```python
from build123d import *

# Parameters (mm, degrees)
SKETCH1_W            = 93
SKETCH1_H            = 100
BOSS_EXTRUDE2_DEPTH  = 10
SKETCH4_W            = 10.01
SKETCH4_H            = 15
BOSS_EXTRUDE4_DEPTH  = 24
SKETCH5_R            = 2
CUT_EXTRUDE1_DEPTH   = 50
SKETCH7_R            = 11
CUT_EXTRUDE3_DEPTH   = 50
SKETCH14_W           = 61.5
SKETCH14_H           = 42
CUT_EXTRUDE8_DEPTH   = 4
SKETCH19_R           = 11
CUT_EXTRUDE11_DEPTH  = 15
SKETCH20_R           = 2
CUT_EXTRUDE12_DEPTH  = 10
SKETCH21_W           = 40
SKETCH21_H           = 6
BOSS_EXTRUDE5_DEPTH  = 27
SKETCH22_W           = 40
SKETCH22_H           = 6.3
BOSS_EXTRUDE7_DEPTH  = 40
SKETCH23_R           = 8
CUT_EXTRUDE13_DEPTH  = 40
SKETCH24_W           = 118.277817783
SKETCH24_H           = 41.8
CUT_EXTRUDE14_DEPTH  = 40
SKETCH25_W           = 31.5
SKETCH25_H           = 23.2
CUT_EXTRUDE15_DEPTH  = 20
CUT_EXTRUDE18_DEPTH  = 3
SKETCH27_R           = 4.1
SKETCH27_R_2         = 4
CUT_EXTRUDE29_DEPTH  = 3
SKETCH28_W           = 29.5
SKETCH28_H           = 58.2
CUT_EXTRUDE30_DEPTH  = 23
SKETCH29_W           = 32
SKETCH29_H           = 4
CUT_EXTRUDE31_DEPTH  = 23
SKETCH31_W           = 32
SKETCH31_H           = 6
BOSS_EXTRUDE9_DEPTH  = 6.6
SKETCH32_W           = 32
SKETCH32_H           = 6
BOSS_EXTRUDE10_DEPTH = 10
SKETCH33_R           = 2
CUT_EXTRUDE32_DEPTH  = 10
BOSS_EXTRUDE11_START = -32
BOSS_EXTRUDE11_DEPTH = 32
SKETCH35_R           = 3.5
CUT_EXTRUDE33_DEPTH  = 10
SKETCH36_W           = 40
SKETCH36_H           = 6.3
BOSS_EXTRUDE12_DEPTH = 18.8
SKETCH37_W           = 40
SKETCH37_H           = 6
BOSS_EXTRUDE13_DEPTH = 16
SKETCH38_R           = 2
CUT_EXTRUDE34_DEPTH  = 16
BOSS_EXTRUDE14_DEPTH = 40
SKETCH40_R           = 3.5
CUT_EXTRUDE35_DEPTH  = 16
SKETCH41_W           = 16
SKETCH41_H           = 64.8
CUT_EXTRUDE36_DEPTH  = 76
SKETCH42_W           = 20.7
SKETCH42_H           = 6
CUT_EXTRUDE37_DEPTH  = 76
SKETCH43_W           = 10.32098901
SKETCH43_H           = 73.075116481
CUT_EXTRUDE38_DEPTH  = 30
SKETCH44_W           = 2
SKETCH44_H           = 70.783229749
CUT_EXTRUDE39_DEPTH  = 30
SKETCH45_W           = 27.67901099
SKETCH45_H           = 15
CUT_EXTRUDE40_DEPTH  = 30
SKETCH46_W           = 27.67901099
SKETCH46_H           = 2.54
CUT_EXTRUDE41_DEPTH  = 110
SKETCH47_R           = 11
CUT_EXTRUDE42_DEPTH  = 20
BOSS_EXTRUDE16_DEPTH = 2.3


with BuildPart() as part:
    # Sketch1 → Boss-Extrude2 (new body)
    with BuildSketch(Plane.XY):
        with Locations((-29.68705036, 14.928057554)):
            Rectangle(SKETCH1_W, SKETCH1_H)
    extrude(amount=BOSS_EXTRUDE2_DEPTH)

    # Sketch4 → Boss-Extrude4 (add)
    with BuildSketch(Plane(origin=(16.81294964, 0, 0), x_dir=(0, 0, -1), z_dir=(1, 0, 0))):
        with Locations((-4.995, -12.571942446)):
            Rectangle(SKETCH4_W, SKETCH4_H)
    extrude(amount=BOSS_EXTRUDE4_DEPTH)

    # Sketch5 → Cut-Extrude1 (cut)
    with BuildSketch(Plane(origin=(0, -5.071942446, 0), x_dir=(1, 0, 0), z_dir=(0, 1, 0))):
        with Locations(Location((26.81294964, -5, 0), (0, 0, 180))):
            Circle(SKETCH5_R)
    extrude(amount=-CUT_EXTRUDE1_DEPTH, mode=Mode.SUBTRACT)

    # Sketch7 → Cut-Extrude3 (cut)
    with BuildSketch(Plane(origin=(0, 0, 0), x_dir=(-1, 0, 0), z_dir=(0, 0, -1))):
        with Locations((24.18705036, 36.928057554)):
            Circle(SKETCH7_R)
    extrude(amount=-CUT_EXTRUDE3_DEPTH, mode=Mode.SUBTRACT)

    # Sketch14 → Cut-Extrude8 (cut)
    with BuildSketch(Plane.XY.offset(10)):
        with Locations((-13.93705036, 36.789132279)):
            Rectangle(SKETCH14_W, SKETCH14_H)
    extrude(amount=-CUT_EXTRUDE8_DEPTH, mode=Mode.SUBTRACT)

    # Sketch19 → Cut-Extrude11 (cut)
    with BuildSketch(Plane(origin=(0, 0, 0), x_dir=(-1, 0, 0), z_dir=(0, 0, -1))):
        with Locations((53.18705036, 36.928057554)):
            Circle(SKETCH19_R)
    extrude(amount=-CUT_EXTRUDE11_DEPTH, mode=Mode.SUBTRACT)

    # Sketch20 → Cut-Extrude12 (cut)
    with BuildSketch(Plane.XY.offset(6)):
        with Locations((-34.68705036, 50.928057554)):
            Circle(SKETCH20_R)
        with Locations((5.31294964, 50.928057554)):
            Circle(SKETCH20_R)
        with Locations((-34.68705036, 22.928057554)):
            Circle(SKETCH20_R)
        with Locations((5.31294964, 22.928057554)):
            Circle(SKETCH20_R)
    extrude(amount=-CUT_EXTRUDE12_DEPTH, mode=Mode.SUBTRACT)

    # Sketch21 → Boss-Extrude5 (add)
    with BuildSketch(Plane(origin=(0, 0, 0), x_dir=(-1, 0, 0), z_dir=(0, 0, -1))):
        with Locations((56.18705036, 61.928057554)):
            Rectangle(SKETCH21_W, SKETCH21_H)
    extrude(amount=BOSS_EXTRUDE5_DEPTH)

    # Sketch22 → Boss-Extrude7 (add)
    with BuildSketch(Plane.XZ.offset(-58.928057554)):
        with Locations((-56.18705036, -23.85)):
            Rectangle(SKETCH22_W, SKETCH22_H)
    extrude(amount=BOSS_EXTRUDE7_DEPTH)

    # Sketch23 → Cut-Extrude13 (cut)
    with BuildSketch(Plane.XY.offset(10)):
        with Locations((-53.18705036, 36.928057554)):
            Circle(SKETCH23_R)
    extrude(amount=-CUT_EXTRUDE13_DEPTH, mode=Mode.SUBTRACT)

    # Sketch24 → Cut-Extrude14 (cut)
    with BuildSketch(Plane.XY.offset(10)):
        with Locations((-17.048141468, -14.171942446)):
            Rectangle(SKETCH24_W, SKETCH24_H)
    extrude(amount=-CUT_EXTRUDE14_DEPTH, mode=Mode.SUBTRACT)

    # Sketch25 → Cut-Extrude15 (cut)
    with BuildSketch(Plane.XY.offset(10)):
        with Locations((-60.43705036, 18.328057554)):
            Rectangle(SKETCH25_W, SKETCH25_H)
    extrude(amount=-CUT_EXTRUDE15_DEPTH, mode=Mode.SUBTRACT)

    # Sketch26 → Cut-Extrude18 (cut)
    with BuildSketch(Plane.XY.offset(6)):
        with BuildLine():
            Line((14.30212304, 57.789132279), (6.863398886, 57.789132279))
            Line((6.863398886, 57.789132279), (6.863398886, 54.615347499))
            ThreePointArc((6.863398886, 54.615347499), (8.24773413, 53.645968516), (9.108195728, 52.191428892))
            Line((9.108195728, 52.191428892), (14.30212304, 52.191428892))
            Line((14.30212304, 52.191428892), (14.30212304, 57.789132279))
        make_face()
        with BuildLine():
            Line((6.863398886, 19.240767609), (6.863398886, 15.789132279))
            Line((6.863398886, 15.789132279), (14.30212304, 15.789132279))
            Line((14.30212304, 15.789132279), (14.30212304, 20.928057554))
            Line((14.30212304, 20.928057554), (8.777051255, 20.928057554))
            ThreePointArc((8.777051255, 20.928057554), (7.95835451, 19.927752057), (6.863398886, 19.240767609))
        make_face()
        with BuildLine():
            Line((-36.237499605, 57.789132279), (-44.68705036, 57.789132279))
            Line((-44.68705036, 57.789132279), (-44.68705036, 52.191428892))
            Line((-44.68705036, 52.191428892), (-38.482296447, 52.191428892))
            ThreePointArc((-38.482296447, 52.191428892), (-37.621834849, 53.645968516), (-36.237499605, 54.615347499))
            Line((-36.237499605, 54.615347499), (-36.237499605, 57.789132279))
        make_face()
        with BuildLine():
            Line((-44.68705036, 21.664686216), (-44.68705036, 15.789132279))
            Line((-44.68705036, 15.789132279), (-36.237499605, 15.789132279))
            Line((-36.237499605, 15.789132279), (-36.237499605, 19.240767609))
            ThreePointArc((-36.237499605, 19.240767609), (-37.621834849, 20.210146592), (-38.482296447, 21.664686216))
            Line((-38.482296447, 21.664686216), (-44.68705036, 21.664686216))
        make_face()
    extrude(amount=-CUT_EXTRUDE18_DEPTH, mode=Mode.SUBTRACT)

    # Sketch27 → Cut-Extrude29 (cut)
    with BuildSketch(Plane.XY.offset(6)):
        with Locations((5.31294964, 50.928057554)):
            Circle(SKETCH27_R)
        with Locations((5.31294964, 22.928057554)):
            Circle(SKETCH27_R_2)
        with Locations((-34.68705036, 50.928057554)):
            Circle(SKETCH27_R)
        with Locations((-34.68705036, 22.928057554)):
            Circle(SKETCH27_R)
    extrude(amount=-CUT_EXTRUDE29_DEPTH, mode=Mode.SUBTRACT)

    # Sketch28 → Cut-Extrude30 (cut)
    with BuildSketch(Plane(origin=(0, 0, 0), x_dir=(-1, 0, 0), z_dir=(0, 0, -1))):
        with Locations((-2.06294964, 35.828057554)):
            Rectangle(SKETCH28_W, SKETCH28_H)
    extrude(amount=-CUT_EXTRUDE30_DEPTH, mode=Mode.SUBTRACT)

    # Sketch29 → Cut-Extrude31 (cut)
    with BuildSketch(Plane(origin=(0, 15.789132279, 0), x_dir=(1, 0, 0), z_dir=(0, 1, 0))):
        with Locations((-28.68705036, -8)):
            Rectangle(SKETCH29_W, SKETCH29_H)
    extrude(amount=-CUT_EXTRUDE31_DEPTH, mode=Mode.SUBTRACT)

    # Sketch31 → Boss-Extrude9 (add)
    with BuildSketch(Plane.XZ.offset(-6.728057554)):
        with Locations((-28.68705036, 3)):
            Rectangle(SKETCH31_W, SKETCH31_H)
    extrude(amount=BOSS_EXTRUDE9_DEPTH)

    # Sketch32 → Boss-Extrude10 (add)
    with BuildSketch(Plane.XY.offset(6)):
        with Locations((-28.68705036, 3.128057554)):
            Rectangle(SKETCH32_W, SKETCH32_H)
    extrude(amount=BOSS_EXTRUDE10_DEPTH)

    # Sketch33 → Cut-Extrude32 (cut)
    with BuildSketch(Plane(origin=(0, 6.128057554, 0), x_dir=(1, 0, 0), z_dir=(0, 1, 0))):
        with Locations(Location((-37.68705036, -11, 0), (0, 0, 270))):
            Circle(SKETCH33_R)
        with Locations(Location((-19.68705036, -11, 0), (0, 0, 270))):
            Circle(SKETCH33_R)
    extrude(amount=-CUT_EXTRUDE32_DEPTH, mode=Mode.SUBTRACT)

    # Sketch34 → Boss-Extrude11 (add)
    with BuildSketch(Plane(origin=(-12.68705036, 0, 0), x_dir=(0, 0, -1), z_dir=(1, 0, 0)).offset(BOSS_EXTRUDE11_START)):
        Polygon((-16, 6.128057554), (-6, 6.128057554), (-6, 14.058360342), align=None)
    extrude(amount=BOSS_EXTRUDE11_DEPTH)

    # Sketch35 → Cut-Extrude33 (cut)
    with BuildSketch(Plane.XZ.offset(-6.128057554)):
        with Locations((-19.68705036, 11)):
            Circle(SKETCH35_R)
        with Locations((-37.68705036, 11)):
            Circle(SKETCH35_R)
    extrude(amount=-CUT_EXTRUDE33_DEPTH, mode=Mode.SUBTRACT)

    # Sketch36 → Boss-Extrude12 (add)
    with BuildSketch(Plane.XZ.offset(-18.928057554)):
        with Locations((-56.18705036, -23.85)):
            Rectangle(SKETCH36_W, SKETCH36_H)
    extrude(amount=BOSS_EXTRUDE12_DEPTH)

    # Sketch37 → Boss-Extrude13 (add)
    with BuildSketch(Plane.XY.offset(-20.7)):
        with Locations((-56.18705036, 3.128057554)):
            Rectangle(SKETCH37_W, SKETCH37_H)
    extrude(amount=BOSS_EXTRUDE13_DEPTH)

    # Sketch38 → Cut-Extrude34 (cut)
    with BuildSketch(Plane(origin=(0, 6.128057554, 0), x_dir=(1, 0, 0), z_dir=(0, 1, 0))):
        with Locations(Location((-58.18705036, 10.7, 0), (0, 0, 180))):
            Circle(SKETCH38_R)
        with Locations(Location((-45.18705036, 10.7, 0), (0, 0, 180))):
            Circle(SKETCH38_R)
    extrude(amount=-CUT_EXTRUDE34_DEPTH, mode=Mode.SUBTRACT)

    # Sketch39 → Boss-Extrude14 (add)
    with BuildSketch(Plane(origin=(-36.18705036, 0, 0), x_dir=(0, 0, -1), z_dir=(1, 0, 0))):
        Polygon((4.7, 6.128057554), (20.7, 18.878141719), (20.7, 6.128057554), align=None)
    extrude(amount=-BOSS_EXTRUDE14_DEPTH)

    # Sketch40 → Cut-Extrude35 (cut)
    with BuildSketch(Plane.XZ.offset(-6.128057554)):
        with Locations(Location((-45.18705036, -10.7, 0), (0, 0, 270))):
            Circle(SKETCH40_R)
        with Locations(Location((-58.18705036, -10.7, 0), (0, 0, 270))):
            Circle(SKETCH40_R)
    extrude(amount=-CUT_EXTRUDE35_DEPTH, mode=Mode.SUBTRACT)

    # Sketch41 → Cut-Extrude36 (cut)
    with BuildSketch(Plane(origin=(-12.68705036, 0, 0), x_dir=(0, 0, -1), z_dir=(1, 0, 0))):
        with Locations((-8, 32.528057554)):
            Rectangle(SKETCH41_W, SKETCH41_H)
    extrude(amount=-CUT_EXTRUDE36_DEPTH, mode=Mode.SUBTRACT)

    # Sketch42 → Cut-Extrude37 (cut)
    with BuildSketch(Plane(origin=(-36.18705036, 0, 0), x_dir=(0, 0, -1), z_dir=(1, 0, 0))):
        with Locations((10.35, 61.928057554)):
            Rectangle(SKETCH42_W, SKETCH42_H)
    extrude(amount=-CUT_EXTRUDE37_DEPTH, mode=Mode.SUBTRACT)

    # Sketch43 → Cut-Extrude38 (cut)
    with BuildSketch(Plane.XY.offset(-4.7)):
        with Locations((-71.026555855, 36.665615794)):
            Rectangle(SKETCH43_W, SKETCH43_H)
    extrude(amount=-CUT_EXTRUDE38_DEPTH, mode=Mode.SUBTRACT)

    # Sketch44 → Cut-Extrude39 (cut)
    with BuildSketch(Plane.XY.offset(-4.7)):
        with Locations((-37.18705036, 35.519672429)):
            Rectangle(SKETCH44_W, SKETCH44_H)
    extrude(amount=-CUT_EXTRUDE39_DEPTH, mode=Mode.SUBTRACT)

    # Sketch45 → Cut-Extrude40 (cut)
    with BuildSketch(Plane.XY.offset(-20.7)):
        with Locations((-52.026555855, 57.428057554)):
            Rectangle(SKETCH45_W, SKETCH45_H)
    extrude(amount=-CUT_EXTRUDE40_DEPTH, mode=Mode.SUBTRACT)

    # Sketch46 → Cut-Extrude41 (cut)
    with BuildSketch(Plane.XY.offset(-4.7)):
        with Locations((-52.026555855, 1.398057554)):
            Rectangle(SKETCH46_W, SKETCH46_H)
    extrude(amount=-CUT_EXTRUDE41_DEPTH, mode=Mode.SUBTRACT)

    # Sketch47 → Cut-Extrude42 (cut)
    with BuildSketch(Plane.XY.offset(-20.7)):
        with Locations((-53.18705036, 36.928057554)):
            Circle(SKETCH47_R)
    extrude(amount=-CUT_EXTRUDE42_DEPTH, mode=Mode.SUBTRACT)

    # Sketch48 → Boss-Extrude16 (add)
    with BuildSketch(Plane.ZY.offset(65.86606135)):
        Polygon((-27, 49.928057554), (-20.7, 49.928057554), (-20.7, 18.878141719), (-4.7, 6.128057554), (-4.7, 2.668057554), (-27, 2.668057554), align=None)
    extrude(amount=BOSS_EXTRUDE16_DEPTH)


solid = part.part
```
Design review of the part built by this model. Coordinates are the model's own, in mm. A direction names the side the tool comes from. Round coordinates to 2 decimals unless told otherwise and drop trailing zeros. Order: outer loops, then holes, each group sorted by start corner. A loop starts at its lowest first (then second) coordinate and runs counter-clockwise, first axis right, second up. Notation, with made-up numbers: (4, 10) - (39, 10) arc R25 cw to (39, 24) - close; hole circle Ø10 at (27.5, 44). An arc over 180 degrees is marked (long way). One line per question, with ' | ' between items.
Item 1: Take a section at B-B, the plane z = -10.7. Write out the cut boundary in (x, y), then the cut area to 3 significant figures.
Checks:
outline: (-68.17, 2.67) - (-60.19, 2.67) - (-60.19, 6.13) - (-61.69, 6.13) - (-61.69, 10.91) - (-68.17, 10.91) - close; (-56.19, 2.67) - (-47.19, 2.67) - (-47.19, 6.13) - (-48.69, 6.13) - (-48.69, 10.91) - (-54.69, 10.91) - (-54.69, 6.13) - (-56.19, 6.13) - close; (-43.19, 2.67) - (-38.19, 2.67) - (-38.19, 10.91) - (-41.69, 10.91) - (-41.69, 6.13) - (-43.19, 6.13) - close | area: 152 mm²
Item 2: Draft analysis for pull direction X (two halves, no side actions). For faces 1 (the face through (-56.19, 4.42, -10.61)), 2 (the face through (-38.187, 15, -21)), 3 (the face through (-52.97, 12.59, -12.81)), 4 (the face through (-47, 6.128, -12)), state which applies: +X half, -X half, draft (parallel to the pull), parting line (faces both ways), or undercut.
Checks:
face 1: undercut | face 2: +X half | face 3: draft | face 4: undercut
Item 3: Machinability: for faces 5 (the face through (-43.03, 32.71, -23.81)), 6 (the face through (-46, 28, -20.7)), 7 (the face through (-60, 6.128, -12)), which of the approach directions +Z, -Z, +X, -X, +Y, -Y give a long, thin tool a straight path to every point of the face, cutting with its end or side? Answer none if there is none.
Checks:
face 5: +Z, -Z | face 6: +Z, +X, -X, +Y | face 7: +Y
Item 4: Take a section at C-C, the plane y = 29. Write out the cut boundary in (x, z).
Checks:
outline: (-68.17, -27) - (-60.81, -27) - (-60.81, -20.7) - (-68.17, -20.7) - close; (-45.56, -27) - (-38.19, -27) - (-38.19, -20.7) - (-45.56, -20.7) - close
Item 5: For P1, Ø4, axis at y = 38, z = -20, coming from the -X side; P2, Ø4, axis at x = -43.5, z = -15.5, coming from the +Y side; P3, Ø1.5, axis at x = -59.5, y = 19.5, coming from the +Z side; P4, Ø15, axis at x = -60.5, y = 36.5, coming from the +Z side, all flat-tipped, find the tip position at first contact; note any pin that passes through.
Checks:
P1: x = -68.17 | P2: y = 16.33 | P3: z = -20.54 | P4: z = -20.7
Item 6: Wall thickness on line 1 (X direction, y = 10.25, z = -10.7); line 2 (X direction, y = 7.5, z = -8.75); line 3 (Y direction, x = -42.25, z = -10.25): over which ranges is each line inside the solid? List them lowest first. Write a range as [from, to].
Checks:
line 1: [-68.17, -61.69], [-54.69, -48.69], [-41.69, -38.19] | line 2: [-68.17, -61.09], [-55.28, -48.09], [-42.28, -38.19] | line 3: [2.67, 6.13]
Item 7: Take a section at D-D, the plane x = -65.5. Write out the cut boundary in (y, z).
Checks:
outline: (2.67, -27) - (49.93, -27) - (49.93, -20.7) - (18.88, -20.7) - (6.13, -4.7) - (2.67, -4.7) - close
Item 8: Take a section at A-A, the plane x = -55.25. Write out the cut boundary in (y, z), then the cut area to 3 significant figures.
Checks:
outline: (2.67, -27) - (26.12, -27) - (26.12, -20.7) - (18.88, -20.7) - (12.43, -12.6) - (6.13, -12.6) - (6.13, -8.8) - (9.39, -8.8) - (6.13, -4.7) - (2.67, -4.7) - close; (47.73, -27) - (49.93, -27) - (49.93, -20.7) - (47.73, -20.7) - close | area: 301 mm²
